The listing builds one solid part. Answer for the finished solid, in the listing's coordinates (mm). A direction names the side the tool comes from. Give positions to 0.01 mm unless a question says otherwise; leave off trailing zeros. Order: outer loops, then holes, each group sorted by start corner. A loop starts at its lowest first (then second) coordinate and runs counter-clockwise, first axis right, second up. Notation, with made-up numbers: (-19, 62) - (6, 62) arc R24 cw to (6, 93) - close; hole circle Ø3 at (68.5, -40). An arc over 180 degrees is marked (long way). Answer as a JSON object with one key per item and string values. Group by question number.
Q1. Consider line 1 (X direction, y = 35.5, z = 2) (3 decimals); line 2 (Y direction, x = -9.5, z = -10). Determine where each line is inside the solid, lowest interval first.
Q2. Given pin 1 (10 mm diameter, centred on x = -6.5, z = 9, fed in from +Y), flat-ended and moving along its own axis, determine where the tip first touches the part or whether it passes through.
Q3. For faces 5 (the face through (9.525, 2, 0)), 6 (the face through (0, -1, -12.7)), determine the directions among +Z, -Z, +X, -X, +Y, -Y from which every point of the face is accessible in a straight line to the end or side of a thin tool.
Q4. A cutting plane is placed at C-C, the plane x = -6. Give the vertices of the cut face in (y, z) (3 decimals).
Q5. A cutting plane is placed at A-A, the plane y = -75. Give the vertices of the cut face in (x, z) (3 decimals), and give its area (3 significant figures).
Q6. The mould has two halves that part along Z. Classify faces 1 (the face through (-9.525, -1, 0)), 2 (the face through (0, -1, 12.7)), 3 (the face through (0, -1, 9.525)), 4 (the face through (-0.178, -98.245, -11.111)): released by +Z, released by -Z, zero draft, split by the parting line, or undercut.
Q7. A cutting plane is placed at B-B, the plane z = 1.5. Give the vertices of the cut face in (x, y) (3 decimals), and give its area (3 significant figures).
Autodesk Inventor part; units mm, degrees
ref_plane "YZ Plane" through (0, 0, 0) normal (1, 0, 0) x (0, 1, 0)
ref_plane "XZ Plane" through (0, 0, 0) normal (0, 1, 0) x (-1, 0, 0)
ref_plane "XY Plane" through (0, 0, 0) normal (0, 0, 1) x (1, 0, 0)
sketch "Sketch1" plane through (0, 0, 0) normal (0, 1, 0) x (-1, 0, 0)
  line L0 (12.7, 12.7) -> (-12.7, 12.7)
  line L1 (-12.7, 12.7) -> (-12.7, -12.7)
  line L2 (-12.7, -12.7) -> (12.7, -12.7)
  line L3 (12.7, -12.7) -> (12.7, 12.7)
  line L4 (12.7, 12.7) -> (-12.7, -12.7) construction
  line L5 (-12.7, 12.7) -> (12.7, -12.7) construction
  line L6 (9.525, 9.525) -> (-9.525, 9.525)
  line L7 (-9.525, 9.525) -> (-9.525, -9.525)
  line L8 (-9.525, -9.525) -> (9.525, -9.525)
  line L9 (9.525, -9.525) -> (9.525, 9.525)
  line L10 (9.525, 9.525) -> (-9.525, -9.525) construction
  line L11 (-9.525, 9.525) -> (9.525, -9.525) construction
  point P0 (0, 0)
  dimension "d0" = 25.4
  dimension "d1" = 25.4
  dimension "d2" = 3.175
  dimension "d3" = 3.175
extrude "Extrusion1" add sketch "Sketch1" along normal mid plane 203.2
sketch "Sketch2" plane through (-12.7, 101.6, 12.7) normal (0, 0, 1) x (1, 0, 0)
  line L0 (25.4, -203.2) -> (0, -203.2)
  line L1 (0, -203.2) -> (25.4, -196.3941)
  line L2 (25.4, -203.2) -> (0, -203.2)
  line L3 (25.4, 0) -> (25.4, -203.2)
  line L4 (25.4, -203.2) -> (25.4, -196.3941)
  point P0 (12.7, -101.6)
  dimension "d6" = 15
extrude "Extrusion2" cut sketch "Sketch2" against normal through all
properties part number "motorBracket-15-degreeBase"
Reply:
{
 "1": {"line 1": "x = -12.7 to -9.525, 9.525 to 12.7", "line 2": "y = -100.74 to 101.6"},
 "2": {"pin 1": "stops at y = 101.6"},
 "3": {"face 5": "+Y, -Y", "face 6": "-Z, +X, -X, +Y, -Y"},
 "4": {"outline": "(-99.805, -12.7) - (101.6, -12.7) - (101.6, -9.525) - (-99.805, -9.525) - close; (-99.805, 9.525) - (101.6, 9.525) - (101.6, 12.7) - (-99.805, 12.7) - close"},
 "5": {"outline": "(-12.7, -12.7) - (12.7, -12.7) - (12.7, 12.7) - (-12.7, 12.7) - close; hole (-9.525, -9.525) - (9.525, -9.525) - (9.525, 9.525) - (-9.525, 9.525) - close", "area": "282 mm^2"},
 "6": {"face 1": "undercut", "face 2": "released by +Z", "face 3": "undercut", "face 4": "zero draft"},
 "7": {"outline": "(-12.7, -101.6) - (-9.525, -100.749) - (-9.525, 101.6) - (-12.7, 101.6) - close; (9.525, -95.645) - (12.7, -94.794) - (12.7, 101.6) - (9.525, 101.6) - close", "area": "1,270 mm^2"}
}
